Autodesk Inventor part; units mm, degrees
ref_plane "YZ Plane" through (0, 0, 0) normal (1, 0, 0) x (0, 1, 0)
ref_plane "XZ Plane" through (0, 0, 0) normal (0, 1, 0) x (-1, 0, 0)
ref_plane "XY Plane" through (0, 0, 0) normal (0, 0, 1) x (1, 0, 0)
sketch "Эскиз1" plane through (0, 0, 0) normal (0, 1, 0) x (-1, 0, 0)
  line L0 (34.2947, -76.014) -> (76.014, -34.2947)
  arc A0 (83.085, -34.2947) -> (76.014, -34.2947) centre (79.5495, -37.8302) ccw
  line L1 (83.085, -34.2947) -> (87.156, -38.3657)
  line L2 (46.3155, -73.8927) -> (73.8927, -46.3155)
  arc A1 (85.2064, -46.3155) -> (73.8927, -46.3155) centre (79.5495, -51.9723) ccw
  line L3 (85.2064, -46.3155) -> (87.5645, -48.6736)
  line L4 (92.5543, -49.5852) -> (94.5192, -45.7288)
  line L5 (87.156, -38.3657) -> (94.5192, -45.7288)
  line L6 (34.2947, -83.085) -> (38.3657, -87.156)
  arc A2 (34.2947, -76.014) -> (34.2947, -83.085) centre (37.8302, -79.5495) ccw
  arc A3 (46.3155, -73.8927) -> (46.3155, -85.2064) centre (51.9723, -79.5495) ccw
  line L7 (48.6736, -87.5645) -> (46.3155, -85.2064)
  line L8 (48.7014, -93.0224) -> (45.7288, -94.5192)
  line L9 (38.3657, -87.156) -> (45.7288, -94.5192)
  spline S0 degree 4 poles (87.5645, -48.6736) (88.1327, -49.2418) (88.8708, -49.8865) (89.7495, -50.471) (90.7127, -50.7263) (91.4939, -50.6999) (92.0261, -50.3682) (92.3519, -49.9478) (92.5543, -49.5852) knots 0 0 0 0 0 0.3763 0.501335 0.614666 0.722287 1 1 1 1 1
  spline S1 degree 4 poles (48.6736, -87.5645) (49.2196, -88.1111) (49.8318, -88.8375) (50.3553, -89.7359) (50.492, -90.7638) (50.3179, -91.6771) (49.7988, -92.3195) (49.2087, -92.7429) (48.7014, -93.0224) knots 0 0 0 0 0 0.349502 0.469309 0.582088 0.694155 1 1 1 1 1
  point P0 (0, 0)
  point P1 (49.5385, -88.5397)
  point P2 (50.0866, -89.3893)
  point P3 (50.374, -90.1304)
  point P4 (50.4468, -90.7861)
  point P5 (50.3313, -91.3833)
  point P6 (50.0252, -91.9468)
  point P7 (49.4982, -92.4922)
  point P8 (88.5759, -49.5937)
  point P9 (89.4338, -50.2024)
  point P10 (90.1559, -50.5529)
  point P11 (90.7644, -50.6948)
  point P12 (91.2858, -50.6665)
  point P13 (91.7467, -50.4838)
  point P14 (92.1672, -50.1352)
extrude "Выдавливание1" add sketch "Эскиз1" along normal blind 35
sketch "Эскиз2" plane through (-73.8927, 0, -46.3155) normal (-0.7071, 0, -0.7071) x (-0.7071, 0, 0.7071)
  line L0 (-39, 0) -> (0, 0) construction
  line L1 (0, 0) -> (0, 35) construction
  line L2 (-39, 35) -> (0, 35) construction
  line L3 (-39, 0) -> (-39, 35) construction
  line L4 (-39, 35) -> (0, 0) construction
  line L5 (0, 0) -> (0, 35) construction
  line L6 (0, 35) -> (-39, 0) construction
  circle A0 centre (-19.5, 17.5) radius 10.3
  circle A1 centre (-19.5, 17.5) radius 7.5 construction
  line L7 (-19.5, 0) -> (-19.5, 35) construction
  circle A2 centre (-19.5, 25) radius 1.25
  circle A3 centre (-25.9952, 21.25) radius 1.25
  circle A4 centre (-25.9952, 13.75) radius 1.25
  circle A5 centre (-19.5, 10) radius 1.25
  circle A6 centre (-13.0048, 13.75) radius 1.25
  circle A7 centre (-13.0048, 21.25) radius 1.25
  circle A8 centre (-19.5, 17.5) radius 5.5
  dimension "d3" = 15
  dimension "d2" = 20.6
  dimension "d4" = 2.5
  dimension "d7" = 360
  dimension "d9" = 11
sketch "Эскиз3" plane through (0, 35, 0) normal (0, 1, 0) x (1, 0, 0)
  arc A0 (-83.085, 34.2947) -> (-76.014, 34.2947) centre (-79.5495, 37.8302) ccw construction
  arc A1 (-34.2947, 76.014) -> (-34.2947, 83.085) centre (-37.8302, 79.5495) ccw construction
  circle A2 centre (-79.5495, 37.8302) radius 2
  circle A3 centre (-37.8302, 79.5495) radius 2
  point P0 (0, 0)
  dimension "d17" = 4
  dimension "d18" = 4
extrude "Выдавливание4" cut sketch "Эскиз3" against normal blind 3.5
sketch "Эскиз4" plane through (0, 0, 0) normal (0, -1, 0) x (1, 0, 0)
  arc A0 (-76.014, -34.2947) -> (-83.085, -34.2947) centre (-79.5495, -37.8302) ccw construction
  arc A1 (-34.2947, -83.085) -> (-34.2947, -76.014) centre (-37.8302, -79.5495) ccw construction
  circle A2 centre (-79.5495, -37.8302) radius 2
  circle A3 centre (-37.8302, -79.5495) radius 2
  point P0 (0, 0)
  dimension "d21" = 4
  dimension "d22" = 4
extrude "Выдавливание5" cut sketch "Эскиз4" against normal blind 3.5
sketch "Эскиз5" plane through (-34.2947, 0, -76.014) normal (0.7071, 0, 0.7071) x (0.7071, 0, -0.7071)
  line L0 (-59, 0) -> (0, 0) construction
  line L1 (0, 0) -> (0, 35) construction
  line L2 (-59, 35) -> (0, 35) construction
  line L3 (-59, 0) -> (-59, 35) construction
  circle A0 centre (-29.5, 12) radius 5.5
  circle A1 centre (-29.5, 12) radius 7.5 construction
  circle A2 centre (-29.5, 12) radius 10.3
  circle A3 centre (-29.5, 19.5) radius 1.25
  line L4 (-29.5, 12) -> (-29.5, 35) construction
  circle A4 centre (-35.9952, 15.75) radius 1.25
  circle A5 centre (-35.9952, 8.25) radius 1.25
  circle A6 centre (-29.5, 4.5) radius 1.25
  circle A7 centre (-23.0048, 8.25) radius 1.25
  circle A8 centre (-23.0048, 15.75) radius 1.25
  point P0 (-29.5, 0)
  dimension "d30" = 15
  dimension "d29" = 11
  dimension "d31" = 20.6
  dimension "d32" = 2.5
  dimension "d35" = 360
  dimension "d44" = 12
extrude "Выдавливание8" cut sketch "Эскиз5" against normal blind 13.5 contours A0 | A3 | A4 | A5 | A6 | A7 | A8
extrude "Выдавливание9" cut sketch "Эскиз5" against normal blind 3.5
chamfer "Фаска2" distance 0.5 angle 45 6 edges at (-60.988, 19.5, -59.2202) (-65.5808, 15.75, -54.6274) (-65.5808, 8.25, -54.6274) (-60.988, 4.5, -59.2202) (-56.3952, 8.25, -63.813) (-56.3952, 15.75, -63.813)
sketch "Эскиз6" plane through (-34.2947, 0, -76.014) normal (0.7071, 0, 0.7071) x (0.7071, 0, -0.7071)
  circle A0 centre (-29.5, 12) radius 10.3 construction
  point P0 (-29.5, 0)
sketch "Эскиз7" plane through (0, 35, 0) normal (0, 1, 0) x (1, 0, 0)
  circle A0 centre (0, 0) radius 98
  line L0 (-94.5632, 25.7254) -> (-115.7616, 51.7347)
  line L1 (-115.7616, 51.7347) -> (-66.5865, 100.4668)
  line L2 (-66.5865, 100.4668) -> (-28.2113, 101.4476)
  line L3 (-28.2113, 101.4476) -> (-27.0576, 94.1907)
  dimension "d45" = 196
sketch "Эскиз8" plane through (-79.5495, 31.5, -37.8302) normal (0, 1, 0) x (1, 0, 0)
  circle A0 centre (0, 0) radius 2
  circle A1 centre (41.7193, 41.7193) radius 2
  point P0 (79.5495, -37.8302)
extrude "Выдавливание11" cut sketch "Эскиз8" against normal blind 100
properties part number "back_motor_mount" material "Пластмасса, непрозрачная, черная"
Could you check a few things on this model? Use its own coordinates, in mm. Give positions to 0.01 mm unless a question says otherwise; leave off trailing zeros. Loops run counter-clockwise (first coordinate to the right, second up) from the corner with the lowest first, then second, coordinate; pieces in that order, holes last. Notation, with made-up numbers: (-11.5, -38.5) - (27.5, -38.5) arc R19 cw to (27.5, -15.5) - close; hole circle Ø1 at (52, 81). An arc over 180 degrees is marked (long way). Answer in a Markdown table with one row per item. Add a question column.
Q1. For pin 1 (3 mm diameter, centred on x = -37.83, z = -79.55, fed in from -Y); pin 2 (8 mm diameter, centred on y = 7.5, z = -72.5, fed in from -X); pin 3 (4 mm diameter, centred on y = 3.5, z = -65, fed in from +X); pin 4 (3 mm diameter, centred on x = -85, y = 15.5, fed in from -Z), each with a flat end and sliding along its axis, tell me the tip position at first contact or that it passes through.
Q2. If we section it at C-C (x = -86): List the corners of the cut face in (y, z) for me, plus the area to 3 significant figures.
Q3. If we section it at B-B (y = 32): State how many separate pieces and enclosed holes the cut face has, plus the area to 3 significant figures.
Q4. Please list where these lines run through material, in increasing order: L1, parallel to Z at x = -45.5, y = 19.5; L2, parallel to X at y = 16, z = -49; L3, parallel to Y at x = -52, z = -61.5. Write a range as from..to.
Q5. We'd pull the mould along Z, two halves only. Please class faces 1 (the face through (-79.462, 17.255, -43.973)), 2 (the face through (-32.83, 17.26, -79.6)), 3 (the face through (-54.734, 16.595, -62.617)): +Z half, -Z half, draft (parallel to the pull), parting line (faces both ways), or undercut.
Q6. If we section it at A-A (z = -69): List the corners of the cut face in (x, y) for me, plus the area to 3 significant figures.
The answers:
| question | item | result |
|---|---|---|
| 1 | pin 1 | passes through |
| 1 | pin 2 | stops at x = -51.71 |
| 1 | pin 3 | stops at x = -43.31 |
| 1 | pin 4 | stops at z = -47.61 |
| 2 | outline | (0, -47.11) - (35, -47.11) - (35, -37.21) - (0, -37.21) - close |
| 2 | area | 346 mm^2 |
| 3 | separate pieces | 1 |
| 3 | enclosed holes | 2 |
| 3 | area | 683 mm^2 |
| 4 | L1 | z = -94.29..-84.25, -74.85..-64.81 |
| 4 | L2 | x = -92.85..-87.9, -71.21..-62.42 |
| 4 | L3 | y = 0..4.19, 19.81..35 |
| 5 | face 1 | -Z half |
| 5 | face 2 | parting line |
| 5 | face 3 | undercut |
| 6 | outline | (-51.21, 0) - (-41.31, 0) - (-41.31, 35) - (-51.21, 35) - close |
| 6 | area | 346 mm^2 |
